```python
from build123d import *

# Parameters (mm, degrees)
SKETCH1_R           = 2
BOSS_EXTRUDE1_DEPTH = 2
CUT_EXTRUDE1_START  = -2
CUT_EXTRUDE1_DEPTH  = 2
FILLET1_R           = 6
BOSS_EXTRUDE2_DEPTH = 1


# Read off the part's stored shape, not the designer's step: Cut-Extrude1
with BuildPart() as part:
    # Sketch1 → Boss-Extrude1 (new body)
    with BuildSketch(Plane(origin=(0, 0, 0), x_dir=(1, 0, 0), z_dir=(0, 1, 0))):
        with BuildLine():
            Line((-1.03527618, 3.863703305), (-12.940952255, 48.296291314))
            ThreePointArc((-12.940952255, 48.296291314), (0, 50), (12.940952255, 48.296291314))
            Line((12.940952255, 48.296291314), (1.03527618, 3.863703305))
            ThreePointArc((1.03527618, 3.863703305), (0, 4), (-1.03527618, 3.863703305))
        make_face()
        with Locations(Location((0, 42.5, 0), (0, 0, 270))):
            Circle(SKETCH1_R, mode=Mode.SUBTRACT)
    extrude(amount=BOSS_EXTRUDE1_DEPTH)

    # Cut-Extrude1 outline → Cut-Extrude1 (cut)
    with BuildSketch(Plane(origin=(0, 2, 0), x_dir=(1, 0, 0), z_dir=(0, 1, 0)).offset(CUT_EXTRUDE1_START)):
        with BuildLine():
            ThreePointArc((-10.484777097, 39.129720832), (-4.720942194, 44.969397941), (1.785714286, 49.96810207))
            ThreePointArc((1.785714286, 49.96810207), (-5.639908806, 49.680896013), (-12.940952255, 48.296291314))
            Line((-12.940952255, 48.296291314), (-10.484777097, 39.129720832))
        make_face()
    extrude(amount=CUT_EXTRUDE1_DEPTH, mode=Mode.SUBTRACT)

    # Fillet1
    fillet1_edges = [part.edges().sort_by_distance(p)[0] for p in [
        (12.940952255, 1, -48.296291314),
        (-10.484777097, 1, -39.129720832),
        (1.785714286, 1, -49.96810207),
    ]]
    fillet(fillet1_edges, radius=FILLET1_R)

    # Sketch4 → Boss-Extrude2 (add)
    with BuildSketch(Plane.XZ):
        with BuildLine():
            Line((-1.5, -37.5), (1.5, -37.5))
            ThreePointArc((1.5, -37.5), (2, -38), (1.5, -38.5))
            Line((1.5, -38.5), (-1.5, -38.5))
            ThreePointArc((-1.5, -38.5), (-2, -38), (-1.5, -37.5))
        make_face()
    extrude(amount=BOSS_EXTRUDE2_DEPTH)


solid = part.part
```
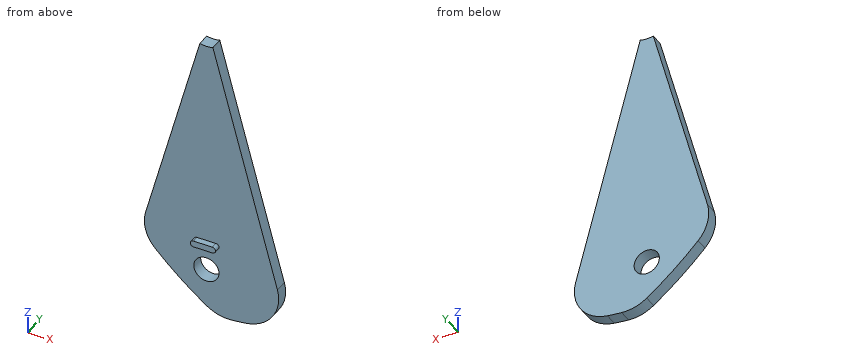
For this review, take the finished solid that the model builds, in its own axes (mm). Round coordinates to 2 decimals unless told otherwise and drop trailing zeros. Write each loop counter-clockwise with the first axis right and the second up, starting at its lowest first coordinate (ties: lowest second). Pieces come first, ordered by that corner, then holes. Notation, with made-up numbers: (-8, -5.5) - (23, -5.5) arc R20 ccw to (23, 2.5) - close; hole circle Ø5 at (78, -10.5). An arc over 180 degrees is marked (long way). Answer as a JSON object with one key per item and string values.
1. For pin 1 Ø1 at (y, z) = (1.5, -27.5) entering from -X; pin 2 Ø1.5 at (x, y) = (8, 0) entering from -Z; pin 3 Ø1.5 at (x, y) = (-7, 0) entering from -Z, all flat-tipped, find the tip position at first contact; note any pin that passes through.
Response values:
{"pin 1": "stops at x = -7.5", "pin 2": "stops at z = -49.39", "pin 3": "stops at z = -43.57"}
2. We need section A-A on z = -38. Give the boundary of the cut face in (x, y).
Response values:
{"outline": "(-9.82, 0) - (-2, 0) - (-2, -1) - (2, -1) - (2, 0) - (10.18, 0) - (10.18, 2) - (-9.82, 2) - close"}
3. To check wall thickness, follow line 1 along Y through (x, z) = (1, -48); line 2 along Z through (x, y) = (1, 1.45); line 3 along Z through (x, y) = (-0.25, 0.9). State the ranges of each line that lie inside material, in increasing order.
Response values:
{"line 1": "y = 0 to 2", "line 2": "z = -49.31 to -44.23, -40.77 to -3.87", "line 3": "z = -48.55 to -44.48, -40.52 to -3.99"}
4. We need section B-B on x = -5.75. Give the boundary of the cut face in (y, z).
Response values:
{"outline": "(0, -44.04) - (2, -44.04) - (2, -21.46) - (0, -21.46) - close"}
5. We need section C-C on x = 10.25. Give the boundary of the cut face in (y, z).
Response values:
{"outline": "(0, -47.3) - (2, -47.3) - (2, -38.25) - (0, -38.25) - close"}
